```python
from build123d import *

# Parameters (mm, degrees)
SKETCH1_W           = 60
SKETCH1_H           = 120
SKETCH1_R           = 1.4
SKETCH1_W_2         = 42
SKETCH1_H_2         = 102
BOSS_EXTRUDE1_DEPTH = 70
SKETCH1_5_W         = 4
SKETCH1_5_H         = 10
BOSS_EXTRUDE3_DEPTH = 60
SKETCH1_7_R         = 1.4
BOSS_EXTRUDE5_DEPTH = 62
SKETCH1_8_R         = 1.4
CUT_EXTRUDE1_DEPTH  = 10
FILLET1_R           = 8


with BuildPart() as part:
    # Sketch1 → Boss-Extrude1 (new body)
    with BuildSketch(Plane.XY):
        with Locations((-17, -25.393258427)):
            Rectangle(SKETCH1_W, SKETCH1_H)
        with Locations((8.5, -25.393258427)):
            Circle(SKETCH1_R, mode=Mode.SUBTRACT)
        with Locations((-42.5, -25.393258427)):
            Circle(SKETCH1_R, mode=Mode.SUBTRACT)
        with Locations((8.5, -80.893258427)):
            Circle(SKETCH1_R, mode=Mode.SUBTRACT)
        with Locations((-42.5, -80.893258427)):
            Circle(SKETCH1_R, mode=Mode.SUBTRACT)
        with Locations((-42.5, 30.106741573)):
            Circle(SKETCH1_R, mode=Mode.SUBTRACT)
        with Locations((8.5, 30.106741573)):
            Circle(SKETCH1_R, mode=Mode.SUBTRACT)
        with Locations((-17, -25.393258427)):
            Rectangle(SKETCH1_W_2, SKETCH1_H_2, mode=Mode.SUBTRACT)
    extrude(amount=-BOSS_EXTRUDE1_DEPTH)

    # Sketch1_5 → Boss-Extrude3 (add)
    with BuildSketch(Plane.XY):
        with Locations((-36, -25.618851522)):
            Rectangle(SKETCH1_5_W, SKETCH1_5_H)
        with Locations((2, -25.618851522)):
            Rectangle(SKETCH1_5_W, SKETCH1_5_H)
    extrude(amount=-BOSS_EXTRUDE3_DEPTH)

    # Sketch1_7 → Boss-Extrude5 (add)
    with BuildSketch(Plane.XY):
        with Locations((8.5, -25.393258427)):
            Circle(SKETCH1_7_R)
        with Locations((-42.5, -25.393258427)):
            Circle(SKETCH1_7_R)
        with Locations((8.5, -80.893258427)):
            Circle(SKETCH1_7_R)
        with Locations((-42.5, -80.893258427)):
            Circle(SKETCH1_7_R)
        with Locations((8.5, 30.106741573)):
            Circle(SKETCH1_7_R)
        with Locations((-42.5, 30.106741573)):
            Circle(SKETCH1_7_R)
    extrude(amount=-BOSS_EXTRUDE5_DEPTH)

    # Sketch1_8 → Cut-Extrude1 (cut)
    with BuildSketch(Plane.XY):
        with Locations((-42.5, -25.393258427)):
            Circle(SKETCH1_8_R)
        with Locations((8.5, -25.393258427)):
            Circle(SKETCH1_8_R)
        with Locations((8.5, 30.106741573)):
            Circle(SKETCH1_8_R)
        with Locations((-42.5, 30.106741573)):
            Circle(SKETCH1_8_R)
        with Locations((8.5, -80.893258427)):
            Circle(SKETCH1_8_R)
        with Locations((-42.5, -80.893258427)):
            Circle(SKETCH1_8_R)
    extrude(amount=-CUT_EXTRUDE1_DEPTH, mode=Mode.SUBTRACT)

    # Fillet1
    fillet1_edges = [part.edges().sort_by_distance(p)[0] for p in [
        (13, -85.393258427, -35),
        (-47, -85.393258427, -35),
        (-47, 34.606741573, -35),
        (13, 34.606741573, -35),
    ]]
    fillet(fillet1_edges, radius=FILLET1_R)


solid = part.part
```
Design review of the part built by this model. Coordinates are the model's own, in mm. A direction names the side the tool comes from. Round coordinates to 2 decimals unless told otherwise and drop trailing zeros. Write each loop counter-clockwise with the first axis right and the second up, starting at its lowest first coordinate (ties: lowest second). Pieces come first, ordered by that corner, then holes. Notation, with made-up numbers: (-27, 25.25) -> (15, 25.25) arc R12 cw to (15, 36.25) -> close; hole circle Ø9 at (-33.5, 10). An arc over 180 degrees is marked (long way). Write item = value, one per line. Start each with the question number.
1) Take a section at B-B, the plane z = -44.5. State the section outline as (x, y) points, plus the area to 3 significant figures.
2) Take a section at D-D, the plane z = -66. State the section outline as (x, y) points, plus the area to 3 significant figures.
3) Clearance check with flat-ended pins moving along their axes: pin 1 (0.8 mm diameter, centred on x = 8.5, y = 30, fed in from -Z); pin 2 (3 mm diameter, centred on x = -42.5, y = 30.11, fed in from -Z); pin 3 (0.8 mm diameter, centred on x = 9, y = -25.5, fed in from +Z). State where each tip first meets the part, or that it passes through.
4) Take a section at C-C, the plane y = -4.5. State the section outline as (x, z) points.
5) Take a section at A-A, the plane x = -13. State the section outline as (y, z) points, plus the area to 3 significant figures.
6) Tool access review of faces 1 (the face through (-47, -26, -35)), 2 (the face through (-36, -26, -60)), 3 (the face through (8.318, 31.495, -4.93)), 4 (the face through (-34, -26, -30)): name each direction out of +Z, -Z, +X, -X, +Y, -Y from which nothing blocks a thin tool from reaching the whole face with its end or side.
7) Mouldability with a two-part tool opening along X and no side actions: class faces 5 (the face through (10.594, -83.112, -35.49)), 6 (the face through (-17, 34.607, -35)), 7 (the face through (-36, -30.619, -30)) as +X half, -X half, draft (parallel to the pull), parting line (faces both ways), or undercut.
8) Wall thickness on probe 1 along Y at (x, z) = (-34.5, -37); probe 2 along Y at (x, z) = (-19, -4); probe 3 along X at (y, z) = (-15.5, -22): over which ranges is each line inside the solid? List them lowest first. Write a range as from..to.
Results list:
q1.outline = (-47, -77.39) arc R8 ccw to (-39, -85.39) -> (5, -85.39) arc R8 ccw to (13, -77.39) -> (13, 26.61) arc R8 ccw to (5, 34.61) -> (-39, 34.61) arc R8 ccw to (-47, 26.61) -> close; hole (-38, -76.39) -> (4, -76.39) -> (4, -30.62) -> (0, -30.62) -> (0, -20.62) -> (4, -20.62) -> (4, 25.61) -> (-38, 25.61) -> (-38, -20.62) -> (-34, -20.62) -> (-34, -30.62) -> (-38, -30.62) -> close
q1.area = 2,940 mm²
q2.outline = (-47, -77.39) arc R8 ccw to (-39, -85.39) -> (5, -85.39) arc R8 ccw to (13, -77.39) -> (13, 26.61) arc R8 ccw to (5, 34.61) -> (-39, 34.61) arc R8 ccw to (-47, 26.61) -> close; hole circle Ø2.8 at (-42.5, -80.89); hole circle Ø2.8 at (-42.5, -25.39); hole circle Ø2.8 at (-42.5, 30.11); hole (-38, -76.39) -> (4, -76.39) -> (4, 25.61) -> (-38, 25.61) -> close; hole circle Ø2.8 at (8.5, -80.89); hole circle Ø2.8 at (8.5, -25.39); hole circle Ø2.8 at (8.5, 30.11)
q2.area = 2,820 mm²
q3.pin_1 = -62
q3.pin_2 = -70
q3.pin_3 = -10
q4.outline = (-47, -70) -> (-38, -70) -> (-38, 0) -> (-47, 0) -> close; (4, -70) -> (13, -70) -> (13, 0) -> (4, 0) -> close
q5.outline = (-85.39, -70) -> (-76.39, -70) -> (-76.39, 0) -> (-85.39, 0) -> close; (25.61, -70) -> (34.61, -70) -> (34.61, 0) -> (25.61, 0) -> close
q5.area = 1,260 mm²
q6.face_1 = +Z, -Z, -X, +Y, -Y
q6.face_2 = -Z
q6.face_3 = +Z
q6.face_4 = +Z, -Z
q7.face_5 = +X half
q7.face_6 = draft
q7.face_7 = undercut
q8.probe_1 = -85.39..-76.39, -30.62..-20.62, 25.61..34.61
q8.probe_2 = -85.39..-76.39, 25.61..34.61
q8.probe_3 = -47..-38, 4..13
